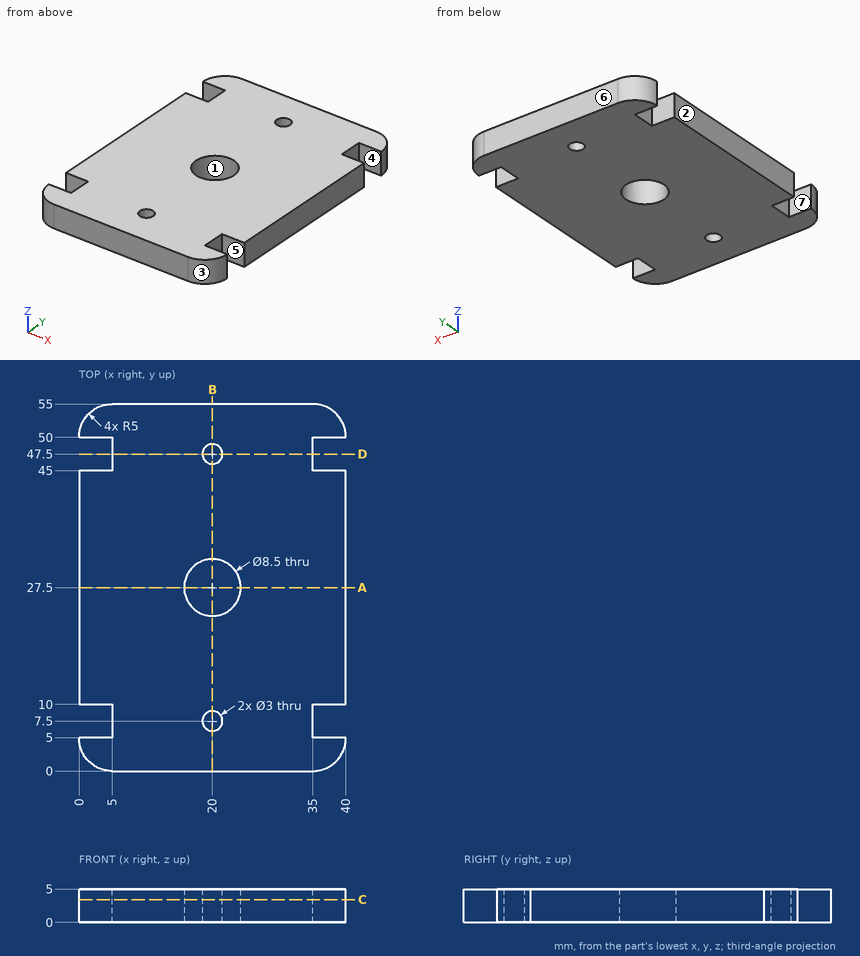
Input: dimensioned drawing with shaded views. Units: mm. Origin: part minimum x, y, z. A direction names the side the tool comes from. Give positions to 0.01 mm unless a question says otherwise; leave off trailing zeros. Write each loop counter-clockwise with the first axis right and the second up, starting at its lowest first coordinate (ties: lowest second). Pieces come first, ordered by that corner, then holes. Notation, with made-up numbers: (-29.5, 82.5) - (-15.5, 82.5) arc R17 ccw to (-15.5, 113.5) - close; hole circle Ø2 at (17, -27.5). An arc over 180 degrees is marked (long way). Write item = value, one per line. Start each with the question number.
1) Material intervals for L1, parallel to Y at x = 20, z = 3.55; L2, parallel to Y at x = 2, z = 1.5; L3, parallel to Y at x = 38.5, z = 3.2, sorted ascending. Write a range as [from, to].
2) Reachability of the marked faces 5, 6 and 7 from +Z, -Z, +X, -X, +Y, -Y: full face, straight path, thin tool, end or side. Return the list, or none.
3) Cut plane D-D (y = 47.5). Return loops of the section in (x, z).
4) Draft query along X for the marked faces 1, 2, 3 and 4. Return one class per face: pulls with the +X half, pulls with the -X half, needs draft (parallel to the pull), parting line crosses it, or undercut.
5) Cut plane B-B (x = 20). Return loops of the section in (y, z).
6) Cut plane A-A (y = 27.5). Return loops of the section in (x, z), and give its area (4 significant figures).
7) Pin query (flat end, axial travel): pin 1 (2.5 mm diameter, centred on x = 37.5, z = 3, fed in from +Y); pin 2 (2.5 mm diameter, centred on x = 37, z = 3.5, fed in from -Y); pin 3 (1.5 mm diameter, centred on x = 3.5, z = 2, fed in from +Y); pin 4 (2.5 mm diameter, centred on x = 20, y = 7.5, fed in from +Z). Return the tip coordinate at first contact, or that it passes through.
8) Cut plane C-C (z = 3.4). Give the number of separate pieces and of enclosed holes in the cut face, and give its area (3 significant figures).
Answers follow:
q1.L1 = [0, 6], [9, 23.25], [31.75, 46], [49, 55]
q1.L2 = [1, 5], [10, 45], [50, 54]
q1.L3 = [1.43, 5], [10, 45], [50, 53.57]
q2.face_5 = +Z, -Z, +X
q2.face_6 = +Z, -Z, +X, -X, +Y
q2.face_7 = +Z, -Z, -X
q3.outline = (5, 0) - (18.5, 0) - (18.5, 5) - (5, 5) - close; (21.5, 0) - (35, 0) - (35, 5) - (21.5, 5) - close
q4.face_1 = undercut
q4.face_2 = pulls with the -X half
q4.face_3 = pulls with the +X half
q4.face_4 = needs draft
q5.outline = (0, 0) - (6, 0) - (6, 5) - (0, 5) - close; (9, 0) - (23.25, 0) - (23.25, 5) - (9, 5) - close; (31.75, 0) - (46, 0) - (46, 5) - (31.75, 5) - close; (49, 0) - (55, 0) - (55, 5) - (49, 5) - close
q6.outline = (0, 0) - (15.75, 0) - (15.75, 5) - (0, 5) - close; (24.25, 0) - (40, 0) - (40, 5) - (24.25, 5) - close
q6.area = 157.5 mm^2
q7.pin_1 = 54.84
q7.pin_2 = 0.06
q7.pin_3 = 54.94
q7.pin_4 = through
q8.separate_pieces = 1
q8.enclosed_holes = 3
q8.area = 2,010 mm^2
